```python
from build123d import *

# Parameters (mm, degrees)
F0_R     = 2.875
F0_R_2   = 3.2
F1_DEPTH = 2.8


with BuildPart() as f1:
    # F0 (on Top) → F1 (new body)
    with BuildSketch(Plane.XY):
        with BuildLine():
            Line((0, -18), (0, 0))
            Line((0, 0), (-28, 0))
            ThreePointArc((-28, 0), (-32.742648, -9), (-28, -18))
            Line((-28, -18), (0, -18))
        make_face()
        with Locations((-8, -12.905)):
            Circle(F0_R, mode=Mode.SUBTRACT)
        with Locations((-28, -9)):
            Circle(F0_R_2, mode=Mode.SUBTRACT)
    extrude(amount=F1_DEPTH)


solid = f1.part
```
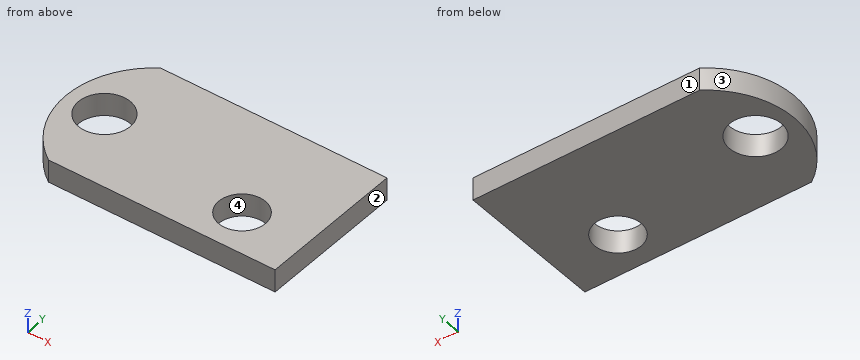
Can you work these out from the model? Positions are in its coordinate system, mm. Face numbers are marked on the shaded views. Round coordinates to 2 decimals unless told otherwise and drop trailing zeros. Order: outer loops, then holes, each group sorted by start corner. A loop starts at its lowest first (then second) coordinate and runs counter-clockwise, first axis right, second up. Notation, with made-up numbers: (50.25, 9) -> (94.25, 9) arc R21 ccw to (94.25, 34) -> close; hole circle Ø7 at (89, 59.25). An arc over 180 degrees is marked (long way). Return JSON: item names as keys, results as strings. Group by question number.
1. Will these pins go through, and if not, where does the flat tip stop? pin 1 (5 mm diameter, centred on x = -28, y = -9, fed in from -Z); pin 2 (1 mm diameter, centred on y = -5, z = 2, fed in from -X).
2. I need wall thicknesses on line 1 (Y direction, x = -8, z = 1.65); line 2 (Y direction, x = -28, z = 2.1); line 3 (X direction, y = -11.5, z = 1.4). Which ranges of each line are inside material? Lowest first, please. Write a range as [from, to].
3. We'd pull the mould along X, two halves only. Please class the marked faces 1, 2, 3 and 4: released by +X, released by -X, zero draft, split by the parting line, or undercut.
4. If we section it at B-B, the plane y = -9: Write out the boundary of the cut face in (x, z).
5. If we section it at D-D, the plane y = -1.5: Write out the boundary of the cut face in (x, z), then the cut area to 3 significant figures.
6. If we section it at C-C, the plane z = 1.95: Write out the boundary of the cut face in (x, y) (3 decimals), then the cut area to 3 significant figures.
7. If we section it at A-A, the plane x = -8: Write out the boundary of the cut face in (y, z).
Output values:
{
 "1": {"pin 1": "through", "pin 2": "x = -32.17"},
 "2": {"line 1": "[-18, -15.78], [-10.03, 0]", "line 2": "[-18, -12.2], [-5.8, 0]", "line 3": "[-32.45, -30], [-26, -10.51], [-5.49, 0]"},
 "3": {"face 1": "zero draft", "face 2": "released by +X", "face 3": "released by -X", "face 4": "undercut"},
 "4": {"outline": "(-32.74, 0) -> (-31.2, 0) -> (-31.2, 2.8) -> (-32.74, 2.8) -> close; (-24.8, 0) -> (0, 0) -> (0, 2.8) -> (-24.8, 2.8) -> close"},
 "5": {"outline": "(-29.76, 0) -> (0, 0) -> (0, 2.8) -> (-29.76, 2.8) -> close", "area": "83.3 mm²"},
 "6": {"outline": "(-28, -18) -> (0, -18) -> (0, 0) -> (-28, 0) arc R10.911 ccw to start; hole circle Ø6.4 at (-28, -9); hole circle Ø5.75 at (-8, -12.905)", "area": "506 mm²"},
 "7": {"outline": "(-18, 0) -> (-15.78, 0) -> (-15.78, 2.8) -> (-18, 2.8) -> close; (-10.03, 0) -> (0, 0) -> (0, 2.8) -> (-10.03, 2.8) -> close"}
}
